```python
from build123d import *

# Parameters (mm, degrees)
BOSS_EXTRUDE1_DEPTH = 2
FILLET1_R           = 2


with BuildPart() as part:
    # Sketch1 → Boss-Extrude1 (new body)
    with BuildSketch(Plane(origin=(0, 0, 0), x_dir=(0, 0, -1), z_dir=(1, 0, 0))):
        Polygon((12.5, 0), (-12.5, 0), (-12.5, 14), (0, 28), (12.5, 14), align=None)
    extrude(amount=BOSS_EXTRUDE1_DEPTH)

    # Fillet1
    fillet1_edges = [part.edges().sort_by_distance(p)[0] for p in [
        (1, 28, 0),
    ]]
    fillet(fillet1_edges, radius=FILLET1_R)


solid = part.part
```
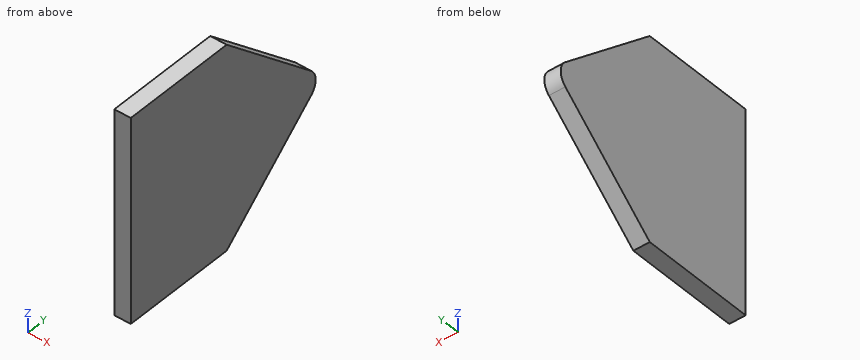
Could you check a few things on this model? Use its own coordinates, in mm. Give positions to 0.01 mm unless a question says otherwise; leave off trailing zeros. Loops run counter-clockwise (first coordinate to the right, second up) from the corner with the lowest first, then second, coordinate; pieces in that order, holes last. Notation, with made-up numbers: (39.25, -37) -> (71.25, -37) arc R38 ccw to (71.25, 1) -> close; hole circle Ø1 at (8.25, 81.5). An arc over 180 degrees is marked (long way). Put each result on its own line as item: value.
(1) Imagine slicing it at C-C on y = 15.5. Write out the boundary of the cut face in (x, z), plus the area to 3 significant figures.
Computed:
outline: (0, -11.16) -> (2, -11.16) -> (2, 11.16) -> (0, 11.16) -> close
area: 44.6 mm^2
(2) Imagine slicing it at A-A on x = 0.65. Write out the boundary of the cut face in (y, z).
Computed:
outline: (0, -12.5) -> (14, -12.5) -> (26.33, -1.49) arc R2 ccw to (26.33, 1.49) -> (14, 12.5) -> (0, 12.5) -> close
(3) I'm going to push a flat-ended pin straight in: pin 1 Ø1 at (x, y) = (1, 17.5) entering from -Z. Where does the tip first touch, or does it pass through?
Computed:
pin 1: z = -9.82
(4) Imagine slicing it at B-B on z = 10.5. Write out the boundary of the cut face in (x, y), plus the area to 3 significant figures.
Computed:
outline: (0, 0) -> (2, 0) -> (2, 16.24) -> (0, 16.24) -> close
area: 32.5 mm^2
(5) Please list where these lines run through material, in increasing order: probe 1 along Z at (x, y) = (1.4, 19.75); probe 2 along Y at (x, z) = (0.4, 8); probe 3 along Z at (x, y) = (1.05, 24.5) (3 decimals). Write a range as [from, to].
Computed:
probe 1: [-7.37, 7.37]
probe 2: [0, 19.04]
probe 3: [-3.125, 3.125]
